Could you check a few things on this model? Use its own coordinates, in mm. A direction names the side the tool comes from. Give positions to 0.01 mm unless a question says otherwise; leave off trailing zeros. Order: outer loops, then holes, each group sorted by start corner. A loop starts at its lowest first (then second) coordinate and runs counter-clockwise, first axis right, second up.
(1) Will these pins go through, and if not, where does the flat tip stop? pin 1 (1.2 mm diameter, centred on y = -118.5, z = 1, fed in from -X); pin 2 (2 mm diameter, centred on x = -15, z = 2, fed in from +Y).
(2) If we mould it in two halves opening along X, with no side actions, what happens to faces 1 (the cylindrical face through (64.694, -74.085, 2.028)), 2 (the flat face through (-43.853, -102, 2)), 3 (the flat face through (-104.36, -68.21, 1.97)), 4 (the cylindrical face through (-2.742, -138.138, 2.028))? For each: released by +X, released by -X, zero draft, split by the parting line, or undercut.
(3) Imagine slicing it at A-A, the plane z = 1.8. State how many separate pieces and enclosed holes the cut face has, then the cut area to 3 significant figures.
(4) Imagine slicing it at C-C, the plane x = -26. Write out the boundary of the cut face in (y, z), then the cut area to 3 significant figures.
(5) Imagine slicing it at B-B, the plane y = -127. Write out the boundary of the cut face in (x, z), then the cut area to 3 significant figures.
(6) On a 3-axis mill with a long thin cutter (end or side, diameter ignored), from which of +Z, -Z, +X, -X, +Y, -Y can I reach the whole of each face in a straight line? I mean faces 5 (the cylindrical face through (-72.458, -74.175, 1.972)), 6 (the flat face through (-24, -76, 0)). Say none if no direction works.
(7) If I drill on probe 1 along X at (y, z) = (-84, 3.8); probe 2 along X at (y, z) = (-86.5, 0.75); probe 3 along X at (y, z) = (-127, 2.1), over which ranges is the centre line in solid material (lowest first)?
from build123d import *

# Parameters (mm, degrees)
SKETCH1_R           = 1.25
BOSS_EXTRUDE1_DEPTH = 4
FILLET1_R           = 2.5
FILLET2_R           = 2.5
FILLET3_R           = 2.5
FILLET4_R           = 2.5
FILLET5_R           = 2.5


with BuildPart() as part:
    # Sketch1 → Boss-Extrude1 (new body)
    with BuildSketch(Plane.XY):
        with BuildLine():
            Line((-99.804604555, -64.168856805), (-111.028493279, -74.119953323))
            Line((-111.028493279, -74.119953323), (-101.028493279, -84.119953323))
            Line((-101.028493279, -84.119953323), (-96.889069885, -88.259376717))
            ThreePointArc((-96.889069885, -88.259376717), (-71.693791888, -73.845522502), (-43.853349067, -65.631451023))
            Line((-43.853349067, -65.631451023), (-43.853349067, -141.295097535))
            ThreePointArc((-43.853349067, -141.295097535), (-34.120648602, -134.791914996), (-22.640145631, -132.508300971))
            ThreePointArc((-22.640145631, -132.508300971), (-11.15964266, -134.791914996), (-1.426942195, -141.295097535))
            Line((-1.426942195, -141.295097535), (-1.426942195, -65.631451023))
            ThreePointArc((-1.426942195, -65.631451023), (26.413500625, -73.845522502), (51.608778623, -88.259376717))
            Line((51.608778623, -88.259376717), (65.748202017, -74.119953323))
            ThreePointArc((65.748202017, -74.119953323), (25.195283415, -47.023359407), (-22.640145631, -37.508300971))
            ThreePointArc((-22.640145631, -37.508300971), (-63.44684459, -44.356647068), (-99.782209189, -64.15128785))
            ThreePointArc((-99.782209189, -64.15128785), (-99.793407372, -64.16007169), (-99.804604555, -64.168856805))
        make_face()
        with BuildLine():
            ThreePointArc((-21.390145631, -122.508300971), (-21.756262155, -123.392184447), (-22.640145631, -123.758300971))
            ThreePointArc((-22.640145631, -123.758300971), (-23.890145631, -122.508300971), (-22.640145631, -121.258300971))
            ThreePointArc((-22.640145631, -121.258300971), (-21.756262155, -121.624417494), (-21.390145631, -122.508300971))
        make_face(mode=Mode.SUBTRACT)
        with Locations((-92.318549214, -71.021033692)):
            Circle(SKETCH1_R, mode=Mode.SUBTRACT)
        with Locations((47.038257951, -71.021033692)):
            Circle(SKETCH1_R, mode=Mode.SUBTRACT)
    extrude(amount=BOSS_EXTRUDE1_DEPTH)

    # Fillet1
    fillet1_edges = [part.edges().sort_by_distance(p)[0] for p in [
        (65.748202017, -74.119953323, 2),
        (51.608778623, -88.259376717, 2),
    ]]
    fillet(fillet1_edges, radius=FILLET1_R)

    # Fillet2
    fillet2_edges = [part.edges().sort_by_distance(p)[0] for p in [
        (-1.426942195, -141.295097535, 2),
        (-43.853349067, -141.295097535, 2),
    ]]
    fillet(fillet2_edges, radius=FILLET2_R)

    # Fillet3
    fillet3_edges = [part.edges().sort_by_distance(p)[0] for p in [
        (-96.889069885, -88.259376717, 2),
        (-111.028493279, -74.119953323, 2),
    ]]
    fillet(fillet3_edges, radius=FILLET3_R)

    # Fillet4
    fillet4_edges = [part.edges().sort_by_distance(p)[0] for p in [
        (-43.853349067, -65.631451023, 2),
    ]]
    fillet(fillet4_edges, radius=FILLET4_R)

    # Fillet5
    fillet5_edges = [part.edges().sort_by_distance(p)[0] for p in [
        (-1.426942195, -65.631451023, 2),
    ]]
    fillet(fillet5_edges, radius=FILLET5_R)


solid = part.part
Answer block:
1. pin 1: stops at x = -43.85
1. pin 2: stops at y = -37.68
2. face 1: released by +X
2. face 2: undercut
2. face 3: released by -X
2. face 4: undercut
3. separate pieces: 1
3. enclosed holes: 3
3. area: 7,260 mm2
4. outline: (-132.7, 0) - (-37.55, 0) - (-37.55, 4) - (-132.7, 4) - close
4. area: 381 mm2
5. outline: (-43.85, 0) - (-1.43, 0) - (-1.43, 4) - (-43.85, 4) - close
5. area: 170 mm2
6. face 5: +Z, -Z, -Y
6. face 6: -Z, +X, -X, +Y, -Y
7. probe 1: x = -101.15 to -90.74, -43.85 to -1.43, 45.46 to 55.87
7. probe 2: x = -98.65 to -94.45, -43.85 to -1.43, 49.16 to 53.37
7. probe 3: x = -43.85 to -1.43
